Geometry check sheet. Reference: the model listing, model coordinates, mm. A direction names the side the tool comes from. Give positions to 0.01 mm unless a question says otherwise; leave off trailing zeros. Loops run counter-clockwise (first coordinate to the right, second up) from the corner with the lowest first, then second, coordinate; pieces in that order, holes last. Notation, with made-up numbers: (16, 32.5) -> (73, 32.5) arc R16 cw to (73, 47.5) -> close; hole circle Ø10 at (17.25, 74). An arc over 180 degrees is marked (long way). Write item = value, one per line.
Autodesk Inventor part; units mm, degrees
ref_plane "WP_H" through (0, 0, 0) normal (0, -1, 0) x (1, 0, 0)
ref_plane "WP_End" through (0, 0, -73.4219) normal (0, 0, -1) x (-1, 0, 0)
sketch "Sketch1" plane through (0, 0, 0) normal (0, 0, 1) x (1, 0, 0)
  line L0 (0, -22.225) -> (0, 22.225) construction
  line L1 (-22.225, 0) -> (22.225, 0) construction
  circle A0 centre (0, 0) radius 15.875
  dimension "d0" = 31.75
extrude "Extrusion1" add sketch "Sketch1" along normal mid plane 48.4188
sketch "Sketch2" plane through (0, 0, 24.2094) normal (0, 0, 1) x (1, 0, 0)
  line L0 (0, -22.2499) -> (0, 22.3742) construction
  line L1 (-22.225, 0) -> (22.225, 0) construction
  line L2 (3.9497, 15.3758) -> (3.9497, 12.1666)
  line L3 (0, 11.4046) -> (3.1877, 11.4046)
  arc A0 (3.1877, 11.4046) -> (3.9497, 12.1666) centre (3.1877, 12.1666) ccw construction
  arc A1 (3.9497, 15.3758) -> (0, 15.875) centre (0, 0) ccw
  line L4 (-3.9497, 15.3758) -> (-3.9497, 12.1666)
  line L5 (0, 11.4046) -> (-3.1877, 11.4046)
  arc A2 (-3.9497, 12.1666) -> (-3.1877, 11.4046) centre (-3.1877, 12.1666) ccw construction
  arc A3 (0, 15.875) -> (-3.9497, 15.3758) centre (0, 0) ccw
  line L6 (-3.9497, 12.1666) -> (-3.9497, 11.4046)
  line L7 (-3.1877, 11.4046) -> (-3.9497, 11.4046)
  line L8 (3.9497, 12.1666) -> (3.9497, 11.4046)
  line L9 (3.1877, 11.4046) -> (3.9497, 11.4046)
  point P0 (0, -15.875)
  dimension "d4" = 3.9497
  dimension "d5" = 27.2796
  dimension "d6" = 1.524
  dimension "d7" = 15.875
  dimension "d8" = 15.875
extrude "Extrusion2" cut sketch "Sketch2" against normal blind 38.1
sketch "Sketch5" plane through (-3.9497, 11.4046, 24.2094) normal (0, 1, 0) x (1, 0, 0)
  line L0 (7.8994, 38.1) -> (0, 38.1)
  line L1 (0, 0) -> (0, 38.1) construction
  line L2 (7.8994, 38.1) -> (7.8994, 0) construction
  arc A0 (7.8994, 38.1) -> (0, 38.1) centre (3.9497, 38.1) ccw
extrude "Extrusion4" cut sketch "Sketch5" along normal up to surface
fillet "Fillet1" radius 0.762 3 edges at (0, 11.4046, -17.8403) (3.9497, 11.4046, 5.1594) (-3.9497, 11.4046, 5.1594)
sketch "Sketch3" plane through (0, 0, -24.2094) normal (0, 0, -1) x (-1, 0, 0)
  circle A0 centre (0, 0) radius 15.875
extrude "Extrusion3" add sketch "Sketch3" along normal blind 98.425
sketch "Sketch4" plane through (0, 0, 0) normal (1, 0, 0) x (0, 1, 0)
  line L0 (27.178, -56.7214) -> (27.178, -90.1224)
  line L1 (0, -147.2946) -> (0, 24.5491) construction
  line L2 (-24.4856, 0) -> (35.7886, 0) construction
  line L3 (15.875, -122.6344) -> (15.875, -17.8403) construction
  line L4 (15.875, -122.6344) -> (-15.875, -122.6344) construction
  line L5 (18.2753, -24.2094) -> (15.875, -24.2094)
  line L6 (26.416, -55.9594) -> (19.7993, -55.9594)
  line L7 (26.416, -90.8844) -> (19.7993, -90.8844)
  line L8 (15.875, -122.6344) -> (18.2753, -122.6344)
  line L9 (19.0373, -24.9714) -> (19.0373, -55.1974)
  line L10 (19.0373, -91.6464) -> (19.0373, -121.8724)
  line L11 (15.875, -24.2094) -> (15.875, -122.6344)
  arc A0 (19.0373, -55.1974) -> (19.7993, -55.9594) centre (19.7993, -55.1974) ccw
  arc A1 (19.7993, -90.8844) -> (19.0373, -91.6464) centre (19.7993, -91.6464) ccw
  line L12 (27.178, -56.7214) -> (26.416, -55.9594)
  line L13 (27.178, -90.1224) -> (26.416, -90.8844)
  line L14 (19.0373, -24.9714) -> (18.2753, -24.2094)
  line L15 (19.0373, -121.8724) -> (18.2753, -122.6344)
  point P0 (0, 0)
  point P1 (27.178, -55.9594)
  point P2 (27.178, -90.8844)
  point P3 (19.0373, -24.2094)
  point P4 (19.0373, -122.6344)
  dimension "d19" = 27.178
  dimension "d20" = 98.425
  dimension "d22" = 34.925
  dimension "d23" = 31.75
  dimension "d24" = 19.0373
  dimension "d25" = 0.762
  dimension "d26" = 0.762
  dimension "d27" = 0.762
  dimension "d28" = 0.762
  dimension "d29" = 0.762
  dimension "d30" = 0.762
  dimension "d31" = 0.762
  dimension "d32" = 0.762
  dimension "d33" = 0.762
  dimension "d34" = 0.762
revolve "Revolution1" add sketch "Sketch4" angle 360 about axis through (0, 0, -10) along (0, 0, 1)
chamfer "Chamfer1" distance 0.762 angle 45 2 edges at (-9.7292, -12.5443, 24.2094) (12.5443, 9.7292, 24.2094)
ref_plane "WP_H" through (0, 0, 0) normal (0, -1, 0) x (1, 0, 0)
ref_plane "WP_End" through (0, 0, -73.4219) normal (0, 0, -1) x (-1, 0, 0)
equation "\"d0\" = K_"
equation "\"d1\" = L_"
equation "\"d4\" = 0.5 * M_"
equation "\"d8\" = 0.5 * K_"
equation "\"d9\" = O_"
equation "\"K_\" = 31.75"
equation "\"L_\" = 48.41875"
equation "\"N_\" = 27.2796"
equation "\"O_\" = 38.1"
equation "\"M_\" = 7.8994"
equation "\"d3\" = K_"
properties part number "ShaftConfig_B_3.7_7.5.FDA658ECE0FAA460A03A372F46ED1B09"
Item 1: Section check D-D, the plane z = 12. Record the cut outline in (x, y) (3 decimals).
Answer:
outline = (-3.95, 12.167) -> (-3.95, 15.376) arc R15.875 ccw (long way) to (3.95, 15.376) -> (3.95, 12.167) arc R0.762 cw to (3.188, 11.405) -> (-3.188, 11.405) arc R0.762 cw to start
Item 2: Tool access check on faces 1 (the flat face through (0, 0, -122.634)), 2 (the flat face through (0, 0, 24.209)), 3 (the cylindrical face through (8.53, -13.39, -0.71)), 4 (the cylindrical face through (5.718, 18.158, -106.971)), 5 (the flat face through (0, 11.405, 4)). Record the directions out of +Z, -Z, +X, -X, +Y, -Y that give a thin tool (end or side, any length) a straight path to the whole face; none if there is none.
Answer:
face_1 = -Z, +X, -X, +Y, -Y
face_2 = +Z, +X, -X, +Y, -Y
face_3 = +Z
face_4 = -Z
face_5 = +Z, +Y
Item 3: Draft check along X on faces 6 (the flat face through (-20, -2, -90.884)), 7 (the cylindrical face through (8.164, 25.923, -73.656)), 8 (the flat face through (-3.95, 14, 5)). Enter one of: +X half, -X half, draft (parallel to the pull), parting line (faces both ways), or undercut.
Answer:
face_6 = draft
face_7 = parting line
face_8 = undercut
Item 4: Thickness scan on L1, parallel to Z at x = -15, y = -6.5; L2, parallel to Z at x = 0.5, y = 25.5; L3, parallel to Y at x = -1, z = 16.5. Record the ranges inside material, lowest first. Write a range as [from, to].
Answer:
L1 = [-122.63, -24.21]
L2 = [-90.88, -55.96]
L3 = [-15.84, 11.4]
Item 5: Section check C-C, the plane z = -78. Record the cut outline in (x, y).
Answer:
outline = circle Ø54.36 at (0, 0)
Item 6: Gauge pin test, flat ends, axial feed: pin 1 (6 mm diameter, centred on x = -17, z = -100, fed in from -Y); pin 2 (1 mm diameter, centred on y = 14.5, z = 12.5, fed in from +X); pin 3 (4 mm diameter, centred on y = 4, z = -4.5, fed in from +X). Record the tip position at first contact, or that the pin passes through.
Answer:
pin_1 = -12.9
pin_2 = 7.48
pin_3 = 15.75
